Read the model definition and answer for the solid it produces. Units are mm, in the model's axes. A direction names the side the tool comes from. Round coordinates to 2 decimals unless told otherwise and drop trailing zeros. Write each loop counter-clockwise with the first axis right and the second up, starting at its lowest first coordinate (ties: lowest second). Pieces come first, ordered by that corner, then holes. Notation, with made-up numbers: (65, 2) - (86, 2) arc R26 ccw to (86, 41) - close; hole circle Ø7 at (-4, 8.5). An arc over 180 degrees is marked (long way). Answer as CSV lines item,"result". Start each with the question number.
1) Each of these flat-tipped pins is pushed along its axis until it touches: pin 1 (1.5 mm diameter, centred on x = -7, z = 82, fed in from -Y); pin 2 (3.5 mm diameter, centred on x = -2.5, z = -132, fed in from -Y); pin 3 (5.5 mm diameter, centred on x = 1, z = -14.5, fed in from -Y) (3 decimals); pin 4 (3 mm diameter, centred on x = -4, z = -133.5, fed in from -Y). Where does it stop, or does it pass through?
2) Find section A-A on z = -44.5. Determine the outline of the cut face in (x, y) (3 decimals).
3) For a pull along X with two mould halves and no side action, classify faces 4 (the flat face through (-3, 1.588, -137)), 5 (the flat face through (-12.5, 3, -2)), 6 (the flat face through (6, 0, 2)) as +X half, -X half, draft (parallel to the pull), parting line (faces both ways), or undercut.
4) Which of the six approach directions +Z, -Z, +X, -X, +Y, -Y give full straight-line access (tool end or side, diameter ignored) to faces 1 (the flat face through (-2, 1.588, 137)), 2 (the flat face through (0, 3, -150)), 3 (the cylindrical face through (0.1, 1.6, 119.7))?
5) Consider line 1 along X through (y, z) = (3.85, 132); line 2 along Z through (x, y) = (-2.75, 2.5); line 3 along X through (y, z) = (2.75, 79.5). Determine where each line is inside the solid, lowest interval first.
Autodesk Inventor part; units mm, degrees
ref_plane "YZ Plane" through (0, 0, 0) normal (1, 0, 0) x (0, 1, 0)
ref_plane "XZ Plane" through (0, 0, 0) normal (0, 1, 0) x (-1, 0, 0)
ref_plane "XY Plane" through (0, 0, 0) normal (0, 0, 1) x (1, 0, 0)
sketch "Sketch1" plane through (0, 0, 0) normal (0, 1, 0) x (-1, 0, 0)
  line L0 (-5.7, -114) -> (5.7, -114)
  line L1 (5.7, -114) -> (5.7, 114)
  line L2 (5.7, 114) -> (-5.7, 114)
  line L3 (-5.7, 114) -> (-5.7, -114)
  line L4 (-5.7, -114) -> (5.7, 114) construction
  line L5 (5.7, -114) -> (-5.7, 114) construction
  line L6 (-12.5, -150) -> (12.5, -150)
  line L7 (12.5, -150) -> (12.5, 150)
  line L8 (12.5, 150) -> (-12.5, 150)
  line L9 (-12.5, 150) -> (-12.5, -150)
  line L10 (-12.5, -150) -> (12.5, 150) construction
  line L11 (12.5, -150) -> (-12.5, 150) construction
  point P0 (0, 0)
  dimension "d0" = 11.4
  dimension "d1" = 228
  dimension "d2" = 300
  dimension "d3" = 25
extrude "Extrusion1" add sketch "Sketch1" along normal blind 6.35
sketch "Sketch2" plane through (0, 6.35, 0) normal (0, 1, 0) x (1, 0, 0)
  line L0 (5.7, 114) -> (5.7, -114)
  line L1 (5.7, -114) -> (-5.7, -114)
  line L2 (-5.7, -114) -> (-5.7, 114)
  line L3 (-5.7, 114) -> (5.7, 114)
  line L4 (12.5, 150) -> (-12.5, 150)
  line L5 (-12.5, 150) -> (-12.5, -150)
  line L6 (-12.5, -150) -> (12.5, -150)
  line L7 (12.5, -150) -> (12.5, 150)
  point P0 (0, 0)
extrude "Extrusion2" add sketch "Sketch2" against normal blind 3.175 contours L0 L1 L2 L3
sketch "Sketch3" plane through (0, 0, 0) normal (0, -1, 0) x (1, 0, 0)
  line L0 (5.7, 114) -> (5.7, -114)
  line L1 (5.7, -114) -> (-5.7, -114)
  line L2 (-5.7, -114) -> (-5.7, 114)
  line L3 (-5.7, 114) -> (5.7, 114)
  line L4 (12.5, -150) -> (-12.5, -150)
  line L5 (12.5, 150) -> (12.5, -150)
  line L6 (-12.5, 150) -> (12.5, 150)
  line L7 (-12.5, -150) -> (-12.5, 150)
  point P0 (0, 0)
  point P1 (-2.5, -132)
  dimension "d8" = 18
  dimension "d36" = 10
hole "Hole1" at (-2.5, 0, -132) direction (0, 1, 0) diameter 4.134 depth 14.2 tip angle 118
sketch "Sketch4" plane through (0, 0, 0) normal (0, -1, 0) x (1, 0, 0)
  circle A0 centre (-2.5, -132) radius 2.067
  line L0 (5.7, 114) -> (5.7, -114)
  line L1 (5.7, -114) -> (-5.7, -114)
  line L2 (-5.7, -114) -> (-5.7, 114)
  line L3 (-5.7, 114) -> (5.7, 114)
  line L4 (12.5, -150) -> (-12.5, -150)
  line L5 (12.5, 150) -> (12.5, -150)
  line L6 (-12.5, 150) -> (12.5, 150)
  line L7 (-12.5, -150) -> (-12.5, 150)
  line L8 (-5.675, -150) -> (0.675, -150)
  line L9 (0.675, -150) -> (0.675, -124.6)
  line L10 (0.675, -124.6) -> (-5.675, -124.6)
  line L11 (-5.675, -124.6) -> (-5.675, -150)
  line L12 (-2.5, -124.6) -> (-2.5, -132) construction
  point P0 (0, 0)
  dimension "d17" = 6.35
  dimension "d18" = 25.4
extrude "Extrusion3" cut sketch "Sketch4" against normal blind 1.5875 contours L4 L11 L10 L9
fillet "Fillet1" radius 3.175 2 edges at (-5.675, 0.7937, -124.6) (0.675, 0.7937, -124.6)
mirror "Mirror1" about plane through (0, 0, 0) normal (0, 0, 1) of "Hole1", "Extrusion3", "Fillet1"
sketch "Sketch7" plane through (0, 0, 0) normal (0, -1, 0) x (1, 0, 0)
  line L0 (5.7, 114) -> (5.7, -114)
  line L1 (5.7, -114) -> (-5.7, -114)
  line L2 (-5.7, -114) -> (-5.7, 114)
  line L3 (-5.7, 114) -> (5.7, 114)
  line L4 (0.675, 150) -> (0.675, 127.775)
  arc A0 (-5.675, 127.775) -> (0.675, 127.775) centre (-2.5, 127.775) ccw
  line L5 (-5.675, 127.775) -> (-5.675, 150)
  line L6 (-12.5, 150) -> (-5.675, 150)
  line L7 (-12.5, -150) -> (-12.5, 150)
  line L8 (-5.675, -150) -> (-12.5, -150)
  line L9 (-5.675, -150) -> (-5.675, -127.775)
  arc A1 (0.675, -127.775) -> (-5.675, -127.775) centre (-2.5, -127.775) ccw
  line L10 (0.675, -127.775) -> (0.675, -150)
  line L11 (12.5, -150) -> (0.675, -150)
  line L12 (12.5, 150) -> (12.5, -150)
  line L13 (0.675, 150) -> (12.5, 150)
  line L14 (-5.7, 114) -> (5.7, 114)
  arc A2 (5.7, 114) -> (-5.7, 114) centre (0, 114) ccw
  line L15 (-5.7, -114) -> (-5.7, 114)
  arc A3 (-5.7, -114) -> (5.7, -114) centre (0, -114) ccw
  line L16 (5.7, 114) -> (5.7, -114)
  point P0 (0, 0)
extrude "Extrusion5" cut sketch "Sketch7" against normal up to surface (3.175 mm away) contours L3 A2 | A3 L1
equation "\"d0\" = 2 * rubberizedCoating + ScintillatorWidth + 2 * silveringThickness"
equation "\"d1\" = 20 * d0"
equation "\"d4\" = mppcMountDepth"
equation "\"d6\" = 0.5 * mppcMountDepth"
equation "\"silveringThickness\" = 0.2"
equation "\"rubberizedCoating\" = 0.5"
equation "\"mppcMountDepth\" = 6.35"
equation "\"OpticalFiberDiameter\" = 1"
equation "\"OpticalFiberClearence\" = 0.1"
equation "\"ScintillatorEdgeClearence\" = 3"
equation "\"ShallowTrackDepth\" = 1.2"
equation "\"DeepTrackDepth\" = 5.6"
equation "\"FiberEdgeOffsett\" = 5"
equation "\"LoopLargeTrackRatio\" = 1.1"
equation "\"FiberSensorClerence\" = 0.5"
equation "\"MountingScrewOffsett\" = 9"
properties part number "mppcMountClamp" material "Aluminum 6061"
Check values:
1,pin 1,"stops at y = 0"
1,pin 2,"passes through"
1,pin 3,"stops at y = 3.175"
1,pin 4,"stops at y = 1.59"
2,outline,"(-12.5, 0) - (-5.7, 0) - (-5.7, 3.175) - (5.7, 3.175) - (5.7, 0) - (12.5, 0) - (12.5, 6.35) - (-12.5, 6.35) - close"
3,face 4,"undercut"
3,face 5,"-X half"
3,face 6,"draft"
4,face 1,"+Z, -Y"
4,face 2,"-Z, +X, -X, +Y, -Y"
4,face 3,"-Y"
5,line 1,"x = -12.5 to -4.57, -0.43 to 12.5"
5,line 2,"z = -150 to -134.05, -129.95 to -118.99, 118.99 to 129.95, 134.05 to 150"
5,line 3,"x = -12.5 to -5.7, 5.7 to 12.5"
